Work out the finished part from the listing and answer in its coordinate system (mm). A direction names the side the tool comes from. Round coordinates to 2 decimals unless told otherwise and drop trailing zeros. Loops run counter-clockwise (first coordinate to the right, second up) from the corner with the lowest first, then second, coordinate; pieces in that order, holes last. Notation, with made-up numbers: (-5, 14.5) - (3, 14.5) arc R24 ccw to (3, 40.5) - close; hole circle Ø11 at (45, 30.5). An arc over 180 degrees is marked (long way). Answer as CSV lines item,"result". Start each with the question number.
Q1. The mould has two halves that part along X. Classify faces 5 (the face through (22, -1, 0)), 6 (the face through (50, -1, -12)), 7 (the face through (45.8, -0.8, -4)): +X half, -X half, draft (parallel to the pull), parting line (faces both ways), or undercut.
Q2. Section D-D on z = -8.5 is taken. Write down the section's boundary in (x, y), then the cut area to 3 significant figures.
Q3. Section A-A on x = 4.25 is taken. Write down the section's boundary in (y, z).
Q4. Section B-B on z = -3.25 is taken. Write down the section's boundary in (x, y), then the cut area to 3 significant figures.
Q5. Each of these flat-tipped pins is pushed along its axis until it touches: pin 1 Ø2 at (x, y) = (35, 1.5) entering from +Z; pin 2 Ø4 at (x, z) = (4.25, -22.5) entering from +Y; pin 3 Ø1.3 at (y, z) = (2, -7.5) entering from -X. Where does it stop, or does it pass through?
Q6. Section C-C on x = 32.5 is taken. Write down the section's boundary in (y, z), then the cut area to 3 significant figures.
Q7. For faces 1 (the face through (33, 1, -5.9)), 2 (the face through (44.25, -1, -1)), 3 (the face through (44.25, -1, -24)), 4 (the face through (38.3, 1, -8)), determine the directions among +Z, -Z, +X, -X, +Y, -Y from which every point of the face is accessible in a straight line to the end or side of a thin tool.
Q8. Straight lines are drawn through the part: L1, parallel to Z at x = 4.25, y = -0.6; L2, parallel to X at y = -0.85, z = -1.5; L3, parallel to Y at x = 19.5, z = -20. For each, find the intervals that lie inside material, in ascending order. Write a range as [from, to].
Autodesk Inventor part; units mm, degrees
ref_plane "YZ Plane" through (0, 0, 0) normal (1, 0, 0) x (0, 1, 0)
ref_plane "XZ Plane" through (0, 0, 0) normal (0, 1, 0) x (-1, 0, 0)
ref_plane "XY Plane" through (0, 0, 0) normal (0, 0, 1) x (1, 0, 0)
sketch "Sketch1" plane through (0, 0, 0) normal (0, 1, 0) x (-1, 0, 0)
  line L0 (-50, 0) -> (-50, -25)
  line L1 (0, -25) -> (0, 0)
  circle A0 centre (-4.25, -22.5) radius 1.5
  circle A1 centre (-4.25, -2.5) radius 1.5
  arc A2 (-44.25, -22.5) -> (-47.25, -22.5) centre (-45.75, -22.5) ccw
  arc A3 (-47.25, -2.5) -> (-44.25, -2.5) centre (-45.75, -2.5) ccw
  line L2 (0, -12.5) -> (-50, -12.5) construction
  line L3 (-25, -25) -> (-25, 0) construction
  line L4 (-44.25, -22.5) -> (-44.25, -25)
  line L5 (-47.25, -22.5) -> (-47.25, -25)
  line L6 (-44.25, -2.5) -> (-44.25, 0)
  line L7 (-47.25, -2.5) -> (-47.25, 0)
  line L8 (0, 0) -> (-44.25, 0)
  line L9 (-47.25, 0) -> (-50, 0)
  line L10 (-50, -25) -> (-47.25, -25)
  line L11 (-44.25, -25) -> (0, -25)
  dimension "d0" = 50
  dimension "d1" = 25
  dimension "d2" = 3
  dimension "d3" = 3
  dimension "d4" = 3
  dimension "d5" = 3
  dimension "d7" = 41.5
  dimension "d8" = 20
  dimension "d9" = 10
  dimension "d10" = 20.75
extrude "Extrusion1" add sketch "Sketch1" against normal blind 1.6
sketch "Sketch2" plane through (0, 0, 0) normal (0, 1, 0) x (1, 0, 0)
  line L0 (38.3, 5.9) -> (28.1, 5.9)
  line L1 (28.1, 5.9) -> (28.1, 10)
  line L2 (28.1, 10) -> (38.3, 10)
  line L3 (38.3, 10) -> (38.3, 5.9)
  line L4 (44.25, 0) -> (0, 0) construction
  line L5 (50, 25) -> (50, 0) construction
  dimension "d13" = 10.2
  dimension "d14" = 4.1
  dimension "d15" = 5.9
  dimension "d16" = 11.7
extrude "Extrusion2" add sketch "Sketch2" along normal blind 2.6
properties part number "basecam_simpleBCG_32bit_tiny"
Findings:
1,face 5,"draft"
1,face 6,"+X half"
1,face 7,"undercut"
2,outline,"(0, -1.6) - (50, -1.6) - (50, 0) - (38.3, 0) - (38.3, 2.6) - (28.1, 2.6) - (28.1, 0) - (0, 0) - close"
2,area,"107 mm^2"
3,outline,"(-1.6, -25) - (0, -25) - (0, -24) - (-1.6, -24) - close; (-1.6, -21) - (0, -21) - (0, -4) - (-1.6, -4) - close; (-1.6, -1) - (0, -1) - (0, 0) - (-1.6, 0) - close"
4,outline,"(0, -1.6) - (2.95, -1.6) - (2.95, 0) - (0, 0) - close; (5.55, -1.6) - (44.45, -1.6) - (44.45, 0) - (5.55, 0) - close; (47.05, -1.6) - (50, -1.6) - (50, 0) - (47.05, 0) - close"
4,area,"71.7 mm^2"
5,pin 1,"stops at z = -5.9"
5,pin 2,"stops at y = 0"
5,pin 3,"stops at x = 28.1"
6,outline,"(-1.6, -25) - (0, -25) - (0, -10) - (2.6, -10) - (2.6, -5.9) - (0, -5.9) - (0, 0) - (-1.6, 0) - close"
6,area,"50.7 mm^2"
7,face 1,"+Z, +X, -X, +Y"
7,face 2,"+Z, +Y, -Y"
7,face 3,"-Z, +Y, -Y"
7,face 4,"+Z, -Z, +X, +Y"
8,L1,"z = [-25, -24], [-21, -4], [-1, 0]"
8,L2,"x = [0, 3.13], [5.37, 44.25], [47.25, 50]"
8,L3,"y = [-1.6, 0]"
